Study the drawing (mm; zero at the part's minimum x, y, z) and answer. Round coordinates to 2 decimals unless told otherwise and drop trailing zeros. Loops run counter-clockwise (first coordinate to the right, second up) from the corner with the lowest first, then second, coordinate; pieces in that order, holes last. Notation, with made-up numbers: (-1, -7) - (17, -7) arc R14 cw to (17, -1) - close; hole circle Ø8 at (-38, 16.25). An arc over 180 degrees is marked (long way). One line per item, written item: value.
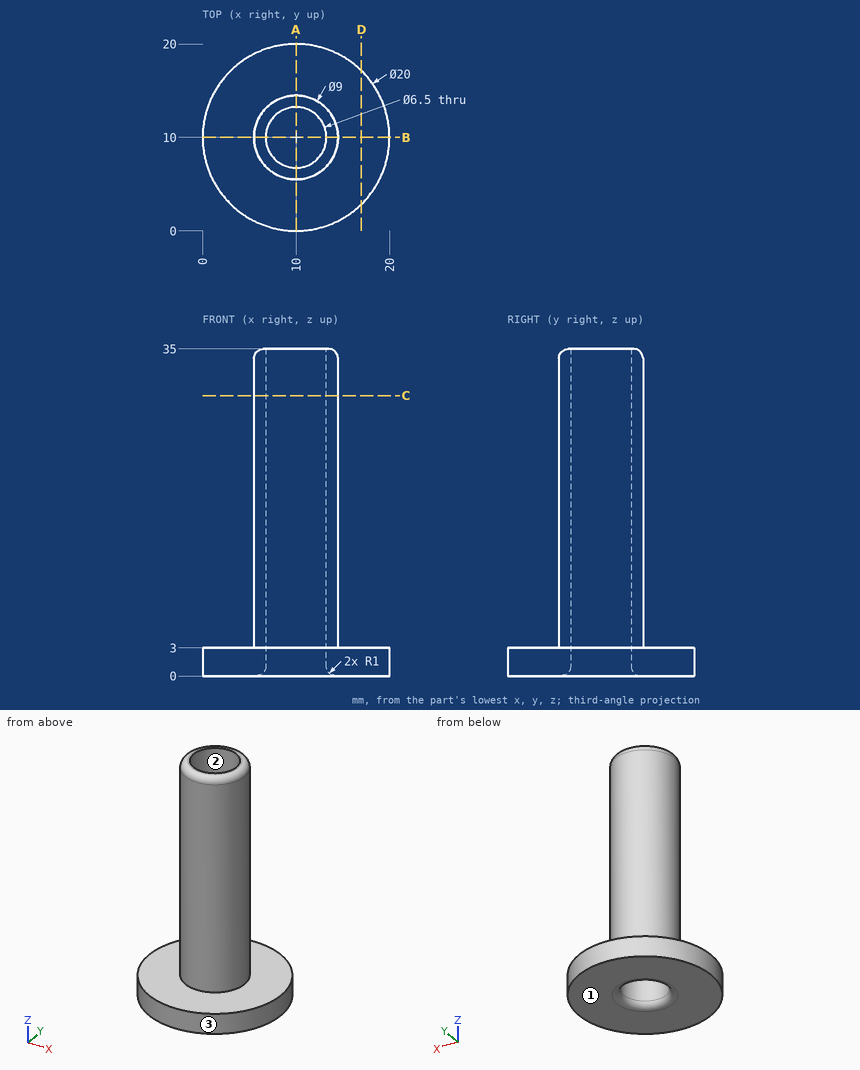
1) A cutting plane is placed at C-C on z = 30. Give the vertices of the cut face in (x, y).
Final values:
outline: circle Ø9 at (10, 10); hole circle Ø6.5 at (10, 10)
2) For a pull along X with two mould halves and no side action, classify the marked faces 1, 2 and 3 as released by +X, released by -X, zero draft, split by the parting line, or undercut.
Final values:
face 1: zero draft
face 2: undercut
face 3: split by the parting line
3) A cutting plane is placed at A-A on x = 10. Give the vertices of the cut face in (y, z).
Final values:
outline: (0, 0) - (5.75, 0) arc R1 ccw to (6.75, 1) - (6.75, 35) - (6.5, 35) arc R1 ccw to (5.5, 34) - (5.5, 3) - (0, 3) - close; (13.25, 1) arc R1 ccw to (14.25, 0) - (20, 0) - (20, 3) - (14.5, 3) - (14.5, 34) arc R1 ccw to (13.5, 35) - (13.25, 35) - close
4) A cutting plane is placed at D-D on x = 17. Give the vertices of the cut face in (y, z), and give its area (3 significant figures).
Final values:
outline: (2.86, 0) - (17.14, 0) - (17.14, 3) - (2.86, 3) - close
area: 42.8 mm2
5) Each of these flat-tipped pins is pushed along its axis until it touches: pin 1 Ø1 at (y, z) = (10, 30) entering from +X; pin 2 Ø10 at (x, z) = (8.5, 11) entering from +Y; pin 3 Ø10.5 at (x, y) = (10, 10) entering from -Z; pin 4 Ø1.5 at (y, z) = (17, 19.5) entering from -X. Where does it stop, or does it pass through?
Final values:
pin 1: x = 14.5
pin 2: y = 14.5
pin 3: z = 0
pin 4: through
6) Consider L1, parallel to Y at x = 10, z = 23; L2, parallel to Z at x = 4.75, y = 9.5; L3, parallel to X at y = 7.5, z = 22.5. Determine where each line is inside the solid, lowest interval first.
Final values:
L1: 5.5 to 6.75, 13.25 to 14.5
L2: 0 to 3
L3: 6.26 to 7.92, 12.08 to 13.74
